Could you check a few things on this model? Use its own coordinates, in mm. Round coordinates to 2 decimals unless told otherwise and drop trailing zeros.
Autodesk Inventor part; units mm, degrees
ref_plane "YZ Plane" through (0, 0, 0) normal (1, 0, 0) x (0, 1, 0)
ref_plane "XZ Plane" through (0, 0, 0) normal (0, 1, 0) x (-1, 0, 0)
ref_plane "XY Plane" through (0, 0, 0) normal (0, 0, 1) x (1, 0, 0)
sketch "Sketch3" plane through (0, 0, 0) normal (0, 0, 1) x (1, 0, 0)
  line L0 (-80.5781, 0.8246) -> (-80.5781, 20.7988) construction
  circle A0 centre (-80.5781, 0.8246) radius 13.481
  line L1 (-53.7179, 12.5571) -> (-53.7179, -10.9927)
  arc A1 (-53.7179, -10.9927) -> (-51.5054, -12.9814) centre (-51.7179, -10.9927) ccw
  arc A2 (-51.5054, 14.5458) -> (-53.7179, 12.5571) centre (-51.7179, 12.5571) ccw
  line L2 (36.2229, -3.6088) -> (-51.5054, -12.9814)
  line L3 (38.0104, 3.1845) -> (38.0104, -1.6201)
  line L4 (-80.5781, 0.8246) -> (49.5525, 0.8246) construction
  circle A3 centre (49.6953, -3.8247) radius 3.848
  line L5 (59.6953, 14.884) -> (59.6953, -12.7998) construction
  spline S0 degree 4 poles (77.9414, 11.0338) (75.5683, 12.9654) (71.7145, 13.0272) (66.8099, 13.9036) (60.7685, 14.7338) (56.2959, 15.3578) (51.7728, 15.9509) (47.2242, 16.5426) (42.6244, 17.1111) (37.9974, 17.6651) (33.3378, 18.1987) (28.6546, 18.7114) (23.9504, 19.2026) (19.2309, 19.6699) (14.5002, 20.1135) (9.7632, 20.5291) (5.025, 20.9191) (0.2903, 21.2792) (-4.4372, 21.6095) (-9.151, 21.9092) (-13.8524, 22.1766) (-18.5268, 22.4102) (-23.2002, 22.6105) (-27.8558, 22.7627) (-32.4748, 22.8704) (-37.0553, 22.9312) (-41.5904, 22.9454) (-46.0738, 22.9127) (-50.5027, 22.8323) (-54.8678, 22.7052) (-59.1755, 22.5324) (-63.394, 22.3084) (-67.5752, 22.0492) (-71.5451, 21.7209) (-75.7777, 21.4072) (-79.04, 20.9063) (-83.4863, 20.5541) (-87.0067, 20.037) (-90.7113, 19.5168) (-94.2172, 18.9459) (-97.6363, 18.3426) (-100.9342, 17.7015) (-104.1216, 17.0263) (-107.1909, 16.3187) (-110.1396, 15.5797) (-112.9656, 14.8117) (-115.6652, 14.0172) (-118.2357, 13.1965) (-120.6759, 12.3541) (-122.9817, 11.4895) (-125.1529, 10.6071) (-127.1857, 9.7065) (-129.0794, 8.7914) (-130.8324, 7.8633) (-132.4429, 6.923) (-133.9096, 5.9737) (-135.2322, 5.016) (-136.4083, 4.0508) (-137.4392, 3.0816) (-138.3215, 2.1025) (-139.0592, 1.1321) (-139.6407, 0.1249) (-140.106, -0.8362) (-140.3589, -2.0477) (-140.602, -2.598) (-140.1166, -5.4607) (-140.0539, -5.4622) (-139.4639, -6.7645) (-138.8842, -7.4979) (-138.1173, -8.3934) (-137.2199, -9.1877) (-136.1721, -9.9852) (-134.9893, -10.738) (-133.6669, -11.4655) (-132.2091, -12.1599) (-130.6156, -12.8245) (-128.8897, -13.4579) (-127.0312, -14.0591) (-125.0439, -14.6296) (-122.9287, -15.1678) (-120.6879, -15.6738) (-118.3241, -16.1476) (-115.8396, -16.5892) (-113.2366, -16.9984) (-110.5176, -17.3742) (-107.6861, -17.7183) (-104.7439, -18.0297) (-101.6943, -18.3095) (-98.5398, -18.5568) (-95.2843, -18.7732) (-91.9297, -18.9579) (-88.48, -19.1131) (-84.9381, -19.2376) (-81.3071, -19.3341) (-77.5906, -19.4015) (-73.7915, -19.4421) (-69.9139, -19.4561) (-65.961, -19.445) (-61.9362, -19.4102) (-57.8434, -19.3518) (-53.6861, -19.2727) (-49.4679, -19.1731) (-45.1932, -19.0538) (-40.8649, -18.9183) (-36.4879, -18.766) (-32.0649, -18.5992) (-27.598, -18.4192) (-23.0941, -18.227) (-18.5434, -18.0273) (-13.9382, -17.8076) (-9.3141, -17.5719) (-4.666, -17.3195) (-0.0002, -17.052) (4.6675, -16.7728) (9.3655, -16.4759) (14.0236, -16.1832) (19.545, -15.7815) (23.3079, -15.6072) (27.1098, -15.1781) (28.8959, -15.0599) knots 0 0 0 0 0 0.024672 0.034555 0.0445 0.054495 0.064543 0.074632 0.084755 0.094911 0.105094 0.115299 0.125521 0.135755 0.145995 0.156237 0.166475 0.176705 0.186921 0.197118 0.207299 0.217463 0.227605 0.23772 0.247796 0.257824 0.267798 0.277713 0.287563 0.297345 0.307053 0.31668 0.326224 0.335555 0.344908 0.354162 0.363308 0.372467 0.381393 0.390196 0.398872 0.407415 0.41582 0.424082 0.432193 0.44015 0.447945 0.455574 0.46303 0.470307 0.477401 0.484305 0.491015 0.497525 0.503831 0.509931 0.515822 0.521506 0.526986 0.53227 0.537373 0.542316 0.547131 0.552525 0.557529 0.562533 0.567581 0.57205 0.576988 0.582082 0.587354 0.592817 0.598478 0.604341 0.610406 0.616671 0.623133 0.629789 0.636632 0.643658 0.650861 0.658236 0.665777 0.673478 0.681333 0.689338 0.697486 0.705771 0.71419 0.722736 0.731403 0.740188 0.749084 0.758087 0.767192 0.776393 0.785687 0.795067 0.804529 0.814069 0.823682 0.833362 0.843106 0.852907 0.862763 0.872667 0.88262 0.892624 0.902675 0.912766 0.92289 0.933033 0.943191 0.953358 0.963531 0.973703 0.984092 1 1 1 1 1
  line L6 (7.5013, -16.4763) -> (50.2906, -13.6435) construction
  arc A4 (44.8353, -17.2546) -> (13.385, -19.3367) centre (31.5327, -54.8885) ccw construction
  line L7 (159.6953, -3.8066) -> (59.6953, -3.8066) construction
  line L8 (-51.5054, 14.5458) -> (36.2229, 5.1732)
  arc A5 (36.2229, -3.6088) -> (38.0104, -1.6201) centre (36.0104, -1.6201) ccw
  arc A6 (38.0104, 3.1845) -> (36.2229, 5.1732) centre (36.0104, 3.1845) ccw
  spline S1 degree 4 poles (78.1029, 11.0141) (76.6463, 11.2227) (73.9909, 10.5042) (70.2765, 8.6041) (66.0429, 5.3938) (62.3889, 1.8499) (60.314, -1.2467) (59.5572, -3.5763) (59.5773, -5.0793) knots 0 0 0 0 0 0.302475 0.43895 0.576633 0.708802 1 1 1 1 1
  spline S2 degree 4 poles (28.8959, -15.0599) (34.0984, -14.7105) (49.269, -14.182) (58.5645, -15.239) (59.5773, -5.0793) knots 0 0 0 0 0 1 1 1 1 1
  line L9 (28.8959, -15.0599) -> (34.0984, -14.7105) construction
  line L10 (34.0984, -14.7105) -> (49.269, -14.182) construction
  line L11 (49.269, -14.182) -> (58.5645, -15.239) construction
  line L12 (58.5645, -15.239) -> (59.5773, -5.0793) construction
  line L13 (-140.4646, -2.8394) -> (159.4818, -3.8173) construction
  line L14 (-132.0856, 0.6333) -> (-132.0856, -6.3667)
  line L15 (-132.0856, -6.3667) -> (-110.3816, -12.3574)
  line L16 (-110.3816, -12.3574) -> (-104.797, -12.3574)
  line L17 (-104.797, -12.3574) -> (-104.797, -18.0156)
  line L18 (-132.0856, 0.6333) -> (-110.3816, 10.553)
  line L19 (-110.3816, 10.553) -> (-104.1736, 10.553)
  line L20 (-104.1736, 10.553) -> (-104.1736, 17.0026)
  line L21 (38.0104, 0.8246) -> (38.0104, -14.6534)
  line L22 (38.0104, 0.8246) -> (38.0104, 17.6585)
  point P0 (0, 0)
  point P1 (17.6589, 23.5628)
  point P2 (75.883, 10.8572)
  point P3 (72.8647, 9.7686)
  point P4 (69.4179, 7.8149)
  point P5 (66.0452, 5.2617)
  point P6 (63.1887, 2.4463)
  point P7 (61.1228, -0.3317)
  point P8 (59.9357, -2.8689)
  point P9 (-160.0931, -3.8671)
  point P10 (28.8959, -15.0599)
  point P11 (69.5533, 13.4647)
  point P12 (65.1899, 14.1023)
  point P13 (60.7936, 14.7318)
  point P14 (56.3207, 15.3468)
  point P15 (51.7945, 15.947)
  point P16 (47.2398, 16.5346)
  point P17 (42.6414, 17.1053)
  point P18 (33.3491, 18.1925)
  point P19 (28.6632, 18.7055)
  point P20 (23.9568, 19.1966)
  point P21 (19.2348, 19.6643)
  point P22 (14.5017, 20.1074)
  point P23 (9.7623, 20.5238)
  point P24 (5.0217, 20.9132)
  point P25 (0.2844, 21.2735)
  point P26 (-4.4451, 21.6038)
  point P27 (-9.1614, 21.9032)
  point P28 (-13.86, 22.1702)
  point P29 (-18.5361, 22.4036)
  point P30 (-23.211, 22.601)
  point P31 (-27.8721, 22.754)
  point P32 (-32.4966, 22.8611)
  point P33 (-37.0797, 22.9217)
  point P34 (-41.6169, 22.9356)
  point P35 (-46.1028, 22.9023)
  point P36 (-50.5329, 22.8216)
  point P37 (-54.9021, 22.6941)
  point P38 (-59.2065, 22.5195)
  point P39 (-63.4406, 22.2977)
  point P40 (-67.6008, 22.0302)
  point P41 (-71.6806, 21.7165)
  point P42 (-75.6814, 21.3591)
  point P43 (-79.1834, 20.9458)
  point P44 (-83.4048, 20.5095)
  point P45 (-87.1309, 20.023)
  point P46 (-90.7527, 19.494)
  point P47 (-94.2725, 18.9266)
  point P48 (-97.6845, 18.3211)
  point P49 (-100.9861, 17.6791)
  point P50 (-107.2438, 16.2934)
  point P51 (-110.1931, 15.553)
  point P52 (-113.0194, 14.7835)
  point P53 (-115.7191, 13.987)
  point P54 (-118.2898, 13.165)
  point P55 (-120.7294, 12.3201)
  point P56 (-123.0349, 11.454)
  point P57 (-125.2048, 10.569)
  point P58 (-127.2364, 9.6666)
  point P59 (-129.1282, 8.7491)
  point P60 (-130.8786, 7.8185)
  point P61 (-132.486, 6.8762)
  point P62 (-133.9488, 5.9245)
  point P63 (-135.2661, 4.9648)
  point P64 (-136.4363, 3.9987)
  point P65 (-137.4592, 3.0275)
  point P66 (-138.3336, 2.0531)
  point P67 (-139.0591, 1.0763)
  point P68 (-139.6352, 0.0983)
  point P69 (-140.0613, -0.8802)
  point P70 (-140.338, -1.8576)
  point P71 (-140.1239, -5.2398)
  point P72 (-139.9547, -5.7022)
  point P73 (-139.492, -6.6066)
  point P74 (-138.8844, -7.4823)
  point P75 (-138.1328, -8.3292)
  point P76 (-137.2384, -9.147)
  point P77 (-136.202, -9.9355)
  point P78 (-135.0249, -10.6943)
  point P79 (-133.7085, -11.4228)
  point P80 (-132.2548, -12.1206)
  point P81 (-130.6648, -12.7879)
  point P82 (-128.941, -13.4239)
  point P83 (-127.0846, -14.0282)
  point P84 (-125.0983, -14.6009)
  point P85 (-122.9839, -15.1415)
  point P86 (-120.7435, -15.6497)
  point P87 (-118.3798, -16.1256)
  point P88 (-115.8952, -16.569)
  point P89 (-113.2918, -16.9797)
  point P90 (-110.5723, -17.3574)
  point P91 (-107.74, -17.7027)
  point P92 (-101.7463, -18.2964)
  point P93 (-98.5909, -18.5451)
  point P94 (-95.3341, -18.7623)
  point P95 (-91.9783, -18.9484)
  point P96 (-88.5271, -19.1041)
  point P97 (-84.9838, -19.2298)
  point P98 (-81.3514, -19.3267)
  point P99 (-77.6332, -19.3951)
  point P100 (-73.8324, -19.4362)
  point P101 (-69.9531, -19.4509)
  point P102 (-65.9985, -19.4404)
  point P103 (-61.9719, -19.4059)
  point P104 (-57.8772, -19.3483)
  point P105 (-53.718, -19.2694)
  point P106 (-49.4979, -19.1701)
  point P107 (-45.2211, -19.0516)
  point P108 (-40.8909, -18.916)
  point P109 (-36.5118, -18.7642)
  point P110 (-32.0871, -18.5977)
  point P111 (-27.6213, -18.418)
  point P112 (-23.1183, -18.2269)
  point P113 (-18.5646, -18.0247)
  point P114 (-13.9566, -17.8054)
  point P115 (-9.3252, -17.5693)
  point P116 (-4.674, -17.317)
  point P117 (-0.0078, -17.05)
  point P118 (4.6686, -16.7695)
  point P119 (9.3513, -16.477)
  point P120 (14.0352, -16.1731)
  point P121 (18.7161, -15.8596)
  point P122 (23.3889, -15.5371)
  point P123 (78.0825, 12.164)
  point P124 (159.2574, -3.8401)
  point P125 (158.8836, -3.8779)
  point P126 (158.3607, -3.9307)
  point P127 (157.6896, -3.9985)
  point P128 (156.8706, -4.081)
  point P129 (155.9046, -4.1779)
  point P130 (154.7931, -4.2892)
  point P131 (153.5367, -4.4143)
  point P132 (152.1372, -4.5532)
  point P133 (150.5955, -4.7056)
  point P134 (148.914, -4.8712)
  point P135 (147.0936, -5.0494)
  point P136 (145.137, -5.2399)
  point P137 (143.0457, -5.4421)
  point P138 (140.8221, -5.6563)
  point P139 (138.4686, -5.8813)
  point P140 (135.9876, -6.1174)
  point P141 (133.3815, -6.3634)
  point P142 (130.6533, -6.6196)
  point P143 (127.8054, -6.8851)
  point P144 (124.8414, -7.1596)
  point P145 (121.7634, -7.4428)
  point P146 (118.5756, -7.7341)
  point P147 (115.2804, -8.0332)
  point P148 (111.8817, -8.3395)
  point P149 (108.3828, -8.6527)
  point P150 (104.787, -8.9722)
  point P151 (101.0985, -9.2974)
  point P152 (97.3206, -9.6283)
  point P153 (93.4572, -9.9643)
  point P154 (89.5122, -10.3048)
  point P155 (85.4898, -10.6492)
  point P156 (81.3936, -10.9969)
  point P157 (77.2284, -11.3479)
  point P158 (72.9975, -11.701)
  point P159 (68.7057, -12.0556)
  point P160 (64.3572, -12.4117)
  point P161 (59.9559, -12.7678)
  point P162 (55.5069, -13.1239)
  point P163 (51.0138, -13.4788)
  point P164 (46.4817, -13.8316)
  point P165 (41.9148, -14.182)
  point P166 (35.7035, -14.3277)
  point P167 (32.6946, -14.8708)
  point P168 (82.2459, 11.5043)
  point P169 (86.3364, 10.8401)
  point P170 (90.3495, 10.1732)
  point P171 (94.2816, 9.5051)
  point P172 (98.1288, 8.837)
  point P173 (101.8872, 8.171)
  point P174 (105.5538, 7.5086)
  point P175 (109.1244, 6.8507)
  point P176 (112.596, 6.1997)
  point P177 (115.9653, 5.5565)
  point P178 (119.2287, 4.9229)
  point P179 (122.3835, 4.3007)
  point P180 (125.4264, 3.6911)
  point P181 (128.3547, 3.0956)
  point P182 (131.1654, 2.5157)
  point P183 (133.8561, 1.9532)
  point P184 (136.4244, 1.4093)
  point P185 (138.8676, 0.8855)
  point P186 (141.1833, 0.383)
  point P187 (143.3697, -0.0964)
  point P188 (145.4247, -0.5518)
  point P189 (147.3462, -0.9817)
  point P190 (149.1327, -1.3852)
  point P191 (150.7821, -1.7608)
  point P192 (152.2935, -2.1073)
  point P193 (153.6651, -2.4241)
  point P194 (154.8954, -2.7103)
  point P195 (155.9838, -2.9647)
  point P196 (156.9291, -3.187)
  point P197 (157.7307, -3.376)
  point P198 (158.3871, -3.5317)
  point P199 (158.8986, -3.6529)
  dimension "d3" = 26.962
  dimension "d6" = 7.696
  dimension "d7" = 110
  dimension "d8" = 100
  dimension "d9" = 2
  dimension "d11" = 4.6493
  dimension "d25" = 7
  dimension "d26" = 3.5
  dimension "d27" = 8.379
  dimension "d28" = 30.083
  dimension "d29" = 5
  dimension "d30" = 5
  dimension "d31" = 59.8865
extrude "Extrusion3" add sketch "Sketch3" along normal blind 74.75 contours L22 S0 S1 S2 L21 L3
properties part number "3P.05.06.JS.flap trailing edge 74_CPY" material "Polyurethane Foam"
Q1. For P1, Ø5, axis at y = 11, z = 33.5, coming from the +X side; P2, Ø12, axis at x = 51.5, z = 48.5, coming from the -Y side; P3, Ø2, axis at x = 63, z = 47, coming from the -Y side, each with a flat end and sliding along its axis, tell me the tip position at first contact or that it passes through.
Q2. We'd pull the mould along Y, two halves only. Please class faces 1 (the cylindrical face through (53.25, -2.35, 36.85)), 2 (the flat face through (53, 2, 0)): released by +Y, released by -Y, zero draft, split by the parting line, or undercut.
Q3. I need wall thicknesses on L1, parallel to Y at x = 49.5, z = 8.5; L2, parallel to X at y = -4, z = 23.5; L3, parallel to Y at x = 52, z = 27.5. Which ranges of each line are inside material? Lowest first, please.
Filled in:
1. P1: stops at x = 77.94
1. P2: stops at y = -14.23
1. P3: stops at y = 0.97
2. face 1: undercut
2. face 2: zero draft
3. L1: y = -13.75 to -7.67, 0.02 to 16.25
3. L2: x = 38.01 to 45.85, 53.54 to 59.66
3. L3: y = -13.23 to -6.91, -0.74 to 15.92
